from build123d import *

# Parameters (mm, degrees)
EXTRUDE_1_DEPTH = 10
EXTRUDE_START   = -10
EXTRUDE_2_DEPTH = 3
SKETCH_2_W      = 20
SKETCH_2_H      = 3
EXTRUDE_3_DEPTH = 20
FILLET_1_R      = 10


with BuildPart() as part:
    # Эскиз1 → Бобышка-Вытянуть1 (new, symmetric)
    with BuildSketch(Plane(origin=(0, 0, 0), x_dir=(1, 0, 0), z_dir=(0, 1, 0))):
        Polygon((20, 0), (0, 0), (0, 20), (3, 20), (3, 3), (20, 3), align=None)
    extrude(amount=EXTRUDE_1_DEPTH, both=True)

    # Эскиз1<3> → Бобышка-Вытянуть2 (add)
    with BuildSketch(Plane(origin=(0, 0, 0), x_dir=(1, 0, 0), z_dir=(0, 1, 0)).offset(EXTRUDE_START)):
        Polygon((3, 20), (20, 3), (3, 3), align=None)
    extrude_2 = extrude(amount=EXTRUDE_2_DEPTH)

    # Зеркальное отражение2: Бобышка-Вытянуть2 across plane
    add(extrude_2.mirror(Plane.ZX))

    # Эскиз2 → Бобышка-Вытянуть3 (add)
    with BuildSketch(Plane(origin=(0, 10, 0), x_dir=(1, 0, 0), z_dir=(0, 1, 0))):
        with Locations((10, 1.5)):
            Rectangle(SKETCH_2_W, SKETCH_2_H)
    extrude(amount=EXTRUDE_3_DEPTH)

    # Скругление1
    fillet_1_edges = [part.edges().sort_by_distance(p)[0] for p in [
        (0, 30, -1.5),
        (20, 30, -1.5),
    ]]
    fillet(fillet_1_edges, radius=FILLET_1_R - 0.0001)  # a hair under: the kernel refuses the full size


solid = part.part
Work out the finished part from the listing and answer in its coordinate system (mm). A direction names the side the tool comes from. Coordinates: 2 decimals unless noted, no trailing zeros. Loops run counter-clockwise (first coordinate to the right, second up) from the corner with the lowest first, then second, coordinate; pieces in that order, holes last. Notation, with made-up numbers: M 73,-33.75 L 102,-33.75 A14 ccw 102,-17.75 Z; hole C 42.5,-29.75 d3. An arc over 180 degrees is marked long. Answer in a Markdown table with one row per item. Add a question column.
1. The mould has two halves that part along Y. Classify faces 1 (the cylindrical face through (17.15, 26.99, -1.52)), 2 (the flat face through (8, 7, -8)), 3 (the flat face through (10, 20, -3)): pulls with the +Y half, pulls with the -Y half, needs draft (parallel to the pull), parting line crosses it, or undercut.
2. Find section D-D, the plane z = -18.5. Write down the section's boundary in (x, y), then the cut area to 3 significant figures.
3. Flat-ended cylindrical pins translate along their axes: P1, Ø4, axis at x = 10.5, y = 24.5, coming from the -Z side; P2, Ø3, axis at x = 17.5, y = 9.5, coming from the -Z side; P3, Ø1, axis at y = 6, z = -8, coming from the +X side. Find the tip coordinate at first contact, or state that the pin passes through.
4. Find section C-C, the plane y = -6. Write down the section's boundary in (x, z).
5. Find section B-B, the plane x = 18.25. Write down the section's boundary in (y, z), then the cut area to 3 significant figures.
6. A tool of negligible diameter and unlimited length cuts with its end or side. For faces 4 (the cylindrical face through (2.85, 26.99, -1.52)), 5 (the flat face through (8, 10, -10)), 6 (the flat face through (8, -7, -8)), from which of +Z, -Z, +X, -X, +Y, -Y can it reach the whole face along a straight path? Write none if from no direction.
7. Find section A-A, the plane z = -16.25. Write down the section's boundary in (x, y), then the cut area to 3 significant figures.
8. Consider L1, parallel to Y at x = 6.5, z = -8.75; L2, parallel to Z at x = 1.25, y = 12; L3, parallel to X at y = 0, z = -5. Determine where each line is inside the solid, lowest interval first.
Reported:
| question | item | result |
|---|---|---|
| 1 | face 1 | pulls with the +Y half |
| 1 | face 2 | undercut |
| 1 | face 3 | needs draft |
| 2 | outline | M 0,-10 L 4.5,-10 L 4.5,-7 L 3,-7 L 3,7 L 4.5,7 L 4.5,10 L 0,10 Z |
| 2 | area | 69.0 mm^2 |
| 3 | P1 | stops at z = -3 |
| 3 | P2 | stops at z = -7 |
| 3 | P3 | stops at x = 3 |
| 4 | outline | M 0,-20 L 3,-20 L 3,-3 L 20,-3 L 20,0 L 0,0 Z |
| 5 | outline | M -10,-4.75 L -7,-4.75 L -7,-3 L 7,-3 L 7,-4.75 L 10,-4.75 L 10,-3 L 25.65,-3 L 25.65,0 L -10,0 Z |
| 5 | area | 117 mm^2 |
| 6 | face 4 | +Z, -Z, -X, +Y |
| 6 | face 5 | -Z, +X, -X, +Y |
| 6 | face 6 | -Z, +X |
| 7 | outline | M 0,-10 L 6.75,-10 L 6.75,-7 L 3,-7 L 3,7 L 6.75,7 L 6.75,10 L 0,10 Z |
| 7 | area | 82.5 mm^2 |
| 8 | L1 | y = -10 to -7, 7 to 10 |
| 8 | L2 | z = -3 to 0 |
| 8 | L3 | x = 0 to 3 |
